Check sheet for the modelled part. Datum: model origin and axes. Units: mm. A direction names the side the tool comes from. Round coordinates to 2 decimals unless told otherwise and drop trailing zeros. Write each loop counter-clockwise with the first axis right and the second up, starting at its lowest first coordinate (ties: lowest second). Pieces come first, ordered by that corner, then holes. Notation, with made-up numbers: (44, 77.5) -> (102, 77.5) arc R17 ccw to (102, 87.5) -> close; hole circle Ø10 at (43, 57.5). An arc over 180 degrees is marked (long way). One line per item, written item: value.
from build123d import *

# Parameters (mm, degrees)
SKETCH1_W                  = 200
SKETCH1_H                  = 54
BOSS_EXTRUDE1_DEPTH        = 75
SHELL1_T                   = 5
BOSS_EXTRUDE2_DEPTH        = 5
BOSS_EXTRUDE3_DEPTH        = 5
SKETCH3_R                  = 1.4
CUT_EXTRUDE1_DEPTH         = 6
BOSS_EXTRUDE4_DEPTH        = 10
SKETCH9_W                  = 45
SKETCH9_H                  = 20
BOSS_EXTRUDE6_DEPTH        = 2
CUT_EXTRUDE2_REACH         = 231.462
SKETCH10_W                 = 12
SKETCH10_H                 = 2
SKETCH11_R                 = 2.3
CUT_EXTRUDE3_DEPTH         = 6
SKETCH13_W                 = 10.5
SKETCH13_H                 = 15
BOSS_EXTRUDE8_DEPTH        = 27
BOSS_EXTRUDE9_DEPTH        = 3.2
CUT_EXTRUDE4_REACH         = 130.496
SKETCH15_R                 = 1.4
CHAMFER8_SIZE              = 0.5
CHAMFER8_OF_MIRROR6_SIZE   = 0.5
CHAMFER3_SIZE              = 40
CHAMFER5_SIZE              = 43
CHAMFER9_SIZE              = 5
CHAMFER10_SIZE             = 2
CHAMFER11_SIZE             = 10
CHAMFER12_SIZE             = 13
CHAMFER13_SIZE             = 4
BOSS_EXTRUDE10_DEPTH       = 3
CHAMFER14_SIZE             = 3
CHAMFER14_OF_MIRROR28_SIZE = 3


# Some blends are built 0.0001 mm under size
with BuildPart() as part:
    # Sketch1 → Boss-Extrude1 (new body)
    with BuildSketch(Plane(origin=(0, 0, 0), x_dir=(1, 0, 0), z_dir=(0, 1, 0))):
        Rectangle(SKETCH1_W, SKETCH1_H)
    extrude(amount=BOSS_EXTRUDE1_DEPTH)

    # Shell1
    shell1_openings = [part.faces().sort_by_distance(p)[0] for p in [
        (0, 75, 0),
    ]]
    offset(amount=SHELL1_T, openings=shell1_openings, kind=Kind.INTERSECTION)

    # Sketch2 → Boss-Extrude2 (add)
    with BuildSketch(Plane(origin=(105, 0, 0), x_dir=(0, 0, -1), z_dir=(1, 0, 0))):
        Polygon((-17, 75), (-6, 86), (6, 86), (17, 75), align=None)
    boss_extrude2 = extrude(amount=-BOSS_EXTRUDE2_DEPTH)

    # Sketch4 → Boss-Extrude3 (add)
    with BuildSketch(Plane(origin=(0, 0, -32), x_dir=(-1, 0, 0), z_dir=(0, 0, -1))):
        Polygon((-80, 75), (-57, 98), (57, 98), (80, 75), align=None)
    boss_extrude3 = extrude(amount=-BOSS_EXTRUDE3_DEPTH)

    # Sketch3 → Cut-Extrude1 (cut)
    with BuildSketch(Plane(origin=(0, 0, -32), x_dir=(-1, 0, 0), z_dir=(0, 0, -1))):
        with Locations((-28, 93)):
            Circle(SKETCH3_R)
        with Locations((-28, 61)):
            Circle(SKETCH3_R)
        with Locations((28, 93)):
            Circle(SKETCH3_R)
        with Locations((28, 61)):
            Circle(SKETCH3_R)
    cut_extrude1 = extrude(amount=-CUT_EXTRUDE1_DEPTH, mode=Mode.SUBTRACT)

    # Mirror4: Boss-Extrude3, Cut-Extrude1 across plane
    add(boss_extrude3.mirror(Plane.XY))
    add(cut_extrude1.mirror(Plane.XY), mode=Mode.SUBTRACT)

    # Mirror5: Boss-Extrude2 across plane
    add(boss_extrude2.mirror(Plane(origin=(0, 0, 0), x_dir=(0, 0, 1), z_dir=(1, 0, 0))))

    # Sketch5 → Boss-Extrude4 (add, symmetric)
    with BuildSketch(Plane.XY):
        Polygon((-100, 75), (-55, 75), (-55, 67), (-100, 22), align=None)
    boss_extrude4 = extrude(amount=BOSS_EXTRUDE4_DEPTH, both=True)

    # Sketch9 → Boss-Extrude6 (add)
    with BuildSketch(Plane(origin=(0, 75, 0), x_dir=(1, 0, 0), z_dir=(0, 1, 0))):
        with Locations((-77.5, 0)):
            Rectangle(SKETCH9_W, SKETCH9_H)
    boss_extrude6 = extrude(amount=BOSS_EXTRUDE6_DEPTH)

    # Sketch10 → Cut-Extrude2 (cut, up to next)
    with BuildSketch(Plane(origin=(-100, 0, 0), x_dir=(0, 0, -1), z_dir=(1, 0, 0)), mode=Mode.PRIVATE) as cut_extrude2_sk1:
        with Locations((0, 76)):
            Rectangle(SKETCH10_W, SKETCH10_H)
    cut_extrude2_tool1 = extrude(cut_extrude2_sk1.sketch, amount=CUT_EXTRUDE2_REACH, mode=Mode.PRIVATE) & part.part
    cut_extrude2 = cut_extrude2_tool1.solids().sort_by_distance((-100, 76, 0))[0]
    add(cut_extrude2, mode=Mode.SUBTRACT)

    # Sketch11 → Cut-Extrude3 (cut)
    with BuildSketch(Plane(origin=(0, 75, 0), x_dir=(1, 0, 0), z_dir=(0, 1, 0))):
        with Locations(Location((-90, 0, 0), (0, 0, 270))):
            Circle(SKETCH11_R)
    cut_extrude3 = extrude(amount=-CUT_EXTRUDE3_DEPTH, mode=Mode.SUBTRACT)

    # Mirror24: Boss-Extrude4, Boss-Extrude6, Cut-Extrude2, Cut-Extrude3 across plane
    add(boss_extrude4.mirror(Plane(origin=(0, 0, 0), x_dir=(0, 0, 1), z_dir=(1, 0, 0))))
    add(boss_extrude6.mirror(Plane(origin=(0, 0, 0), x_dir=(0, 0, 1), z_dir=(1, 0, 0))))
    add(cut_extrude2.mirror(Plane(origin=(0, 0, 0), x_dir=(0, 0, 1), z_dir=(1, 0, 0))), mode=Mode.SUBTRACT)
    add(cut_extrude3.mirror(Plane(origin=(0, 0, 0), x_dir=(0, 0, 1), z_dir=(1, 0, 0))), mode=Mode.SUBTRACT)

    # Sketch13 → Boss-Extrude8 (add, symmetric)
    with BuildSketch(Plane.XY):
        with Locations((35.75, 23.7)):
            Rectangle(SKETCH13_W, SKETCH13_H)
        with Locations((-15.75, 23.7)):
            Rectangle(SKETCH13_W, SKETCH13_H)
    extrude(amount=BOSS_EXTRUDE8_DEPTH, both=True)

    # Sketch14 → Boss-Extrude9 (add)
    with BuildSketch(Plane(origin=(0, 31.2, 0), x_dir=(1, 0, 0), z_dir=(0, 1, 0))):
        with BuildLine():
            Line((-10.5, -27), (-10.5, -9.6))
            Line((-10.5, -9.6), (-15.5, -9.6))
            ThreePointArc((-15.5, -9.6), (-16.914213562, -9.014213562), (-17.5, -7.6))
            Line((-17.5, -7.6), (-17.5, 7.6))
            ThreePointArc((-17.5, 7.6), (-16.914213562, 9.014213562), (-15.5, 9.6))
            Line((-15.5, 9.6), (-10.5, 9.6))
            Line((-10.5, 9.6), (-10.5, 27))
            Line((-10.5, 27), (-21, 27))
            Line((-21, 27), (-21, -27))
            Line((-21, -27), (-10.5, -27))
        make_face()
    boss_extrude9 = extrude(amount=BOSS_EXTRUDE9_DEPTH)

    # Sketch15 → Cut-Extrude4 (cut, up to next)
    with BuildSketch(Plane(origin=(0, 31.2, 0), x_dir=(1, 0, 0), z_dir=(0, 1, 0)), mode=Mode.PRIVATE) as cut_extrude4_sk1:
        with Locations(Location((-14.8, 5, 0), (0, 0, 180))):
            Circle(SKETCH15_R)
    cut_extrude4_tool1 = extrude(cut_extrude4_sk1.sketch, amount=-CUT_EXTRUDE4_REACH, mode=Mode.PRIVATE) & part.part
    # Sketch15 → Cut-Extrude4 (cut, up to next)
    with BuildSketch(Plane(origin=(0, 31.2, 0), x_dir=(1, 0, 0), z_dir=(0, 1, 0)), mode=Mode.PRIVATE) as cut_extrude4_sk2:
        with Locations(Location((-14.8, -5, 0), (0, 0, 180))):
            Circle(SKETCH15_R)
    cut_extrude4_tool2 = extrude(cut_extrude4_sk2.sketch, amount=-CUT_EXTRUDE4_REACH, mode=Mode.PRIVATE) & part.part
    cut_extrude4_1 = cut_extrude4_tool1.solids().sort_by_distance((-14.8, 31.2, -5))[0]
    add(cut_extrude4_1, mode=Mode.SUBTRACT)
    cut_extrude4_2 = cut_extrude4_tool2.solids().sort_by_distance((-14.8, 31.2, 5))[0]
    add(cut_extrude4_2, mode=Mode.SUBTRACT)
    cut_extrude4 = cut_extrude4_1 + cut_extrude4_2  # Cut-Extrude4 as one shape, for the pattern or mirror that repeats it

    # Chamfer8
    chamfer8_edges = [part.edges().sort_by_distance(p)[0] for p in [
        (-13.4, 31.2, -5),
        (-13.4, 31.2, 5),
    ]]
    chamfer(chamfer8_edges, length=CHAMFER8_SIZE)

    # Mirror6: Boss-Extrude9, Cut-Extrude4 across plane
    add(boss_extrude9.mirror(Plane(origin=(10, 0, 0), x_dir=(0, 0, 1), z_dir=(1, 0, 0))))
    add(cut_extrude4.mirror(Plane(origin=(10, 0, 0), x_dir=(0, 0, 1), z_dir=(1, 0, 0))), mode=Mode.SUBTRACT)

    # Chamfer8 of Mirror6
    chamfer8_of_mirror6_edges = [part.edges().sort_by_distance(p)[0] for p in [
        (33.4, 31.2, -5),
        (33.4, 31.2, 5),
    ]]
    chamfer(chamfer8_of_mirror6_edges, length=CHAMFER8_OF_MIRROR6_SIZE)

    # Chamfer3
    # the kernel refuses this chamfer: 40 mm, written as the material it adds along each edge
    with BuildSketch(Plane(origin=(100, 0, 27), x_dir=(0.027495876610586317, 0.9996219169112968, 0), z_dir=(0, 0, -1)), Plane(origin=(-100, 0, -27), x_dir=(-0.027495876610586317, 0.9996219169112968, 0), z_dir=(0, 0, 1))) as chamfer3_piece_1:
        Polygon((CHAMFER3_SIZE * 0.999621916911, -CHAMFER3_SIZE * 0.0274958766106), (-CHAMFER3_SIZE * 0.0274958766106, -CHAMFER3_SIZE * 0.999621916911), (0, 0), align=None)
    extrude(amount=54)

    # Chamfer5
    chamfer5_edges = [part.edges().sort_by_distance(p)[0] for p in [
        (-105, -5, 0),
        (105, -5, 0),
    ]]
    chamfer(chamfer5_edges, length=CHAMFER5_SIZE)

    # Chamfer9
    chamfer9_edges = [part.edges().sort_by_distance(p)[0] for p in [
        (35.75, 16.2, -27),
        (35.75, 16.2, 27),
        (-15.75, 16.2, -27),
        (-15.75, 16.2, 27),
    ]]
    chamfer(chamfer9_edges, length=CHAMFER9_SIZE)

    # Chamfer10
    chamfer10_edges = [part.edges().sort_by_distance(p)[0] for p in [
        (30.5, 22.8, -27),
        (41, 22.8, -27),
        (30.5, 22.8, 27),
        (41, 22.8, 27),
        (-10.5, 22.8, 27),
        (-21, 22.8, 27),
        (-10.5, 22.8, -27),
        (-21, 22.8, -27),
    ]]
    chamfer(chamfer10_edges, length=CHAMFER10_SIZE)

    # Chamfer11
    chamfer11_edges = [part.edges().sort_by_distance(p)[0] for p in [
        (-80, 20, -27),
        (80, 20, -27),
        (-80, 20, 27),
        (80, 20, 27),
    ]]
    chamfer(chamfer11_edges, length=CHAMFER11_SIZE)

    # Chamfer12
    chamfer12_edges = [part.edges().sort_by_distance(p)[0] for p in [
        (-83.5, 16.5, -32),
        (83.5, 16.5, -32),
        (-83.5, 16.5, 32),
        (83.5, 16.5, 32),
    ]]
    chamfer(chamfer12_edges, length=CHAMFER12_SIZE)

    # Chamfer13
    chamfer13_edges = [part.edges().sort_by_distance(p)[0] for p in [
        (-100, 58.5, -10),
        (-100, 58.5, 10),
        (100, 58.5, 10),
        (100, 58.5, -10),
    ]]
    chamfer(chamfer13_edges, length=CHAMFER13_SIZE)

    # Sketch16 → Boss-Extrude10 (add)
    with BuildSketch(Plane(origin=(105, 0, 0), x_dir=(0, 0, -1), z_dir=(1, 0, 0))):
        Polygon((-19, 38), (19, 38), (32, 56.384776311), (32, 75), (17, 75), (6, 86), (-6, 86), (-17, 75), (-32, 75), (-32, 56.384776311), align=None)
    boss_extrude10 = extrude(amount=BOSS_EXTRUDE10_DEPTH)

    # Chamfer14
    chamfer14_edges = [part.edges().sort_by_distance(p)[0] for p in [
        (108, 65.692388155, 32),
        (108, 75, 24.5),
        (108, 80.5, 11.5),
        (108, 86, 0),
        (108, 80.5, -11.5),
        (108, 75, -24.5),
        (108, 65.692388155, -32),
        (108, 47.192388155, -25.5),
        (108, 38, 0),
        (108, 47.192388155, 25.5),
    ]]
    chamfer(chamfer14_edges, length=CHAMFER14_SIZE - 0.0001)  # a hair under: the kernel refuses the full size

    # Mirror28: Boss-Extrude10 across plane
    add(boss_extrude10.mirror(Plane(origin=(0, 0, 0), x_dir=(0, 0, 1), z_dir=(1, 0, 0))))

    # Chamfer14 of Mirror28
    chamfer14_of_mirror28_edges = [part.edges().sort_by_distance(p)[0] for p in [
        (-108, 65.692388155, 32),
        (-108, 75, 24.5),
        (-108, 80.5, 11.5),
        (-108, 86, 0),
        (-108, 80.5, -11.5),
        (-108, 75, -24.5),
        (-108, 65.692388155, -32),
        (-108, 47.192388155, -25.5),
        (-108, 38, 0),
        (-108, 47.192388155, 25.5),
    ]]
    chamfer(chamfer14_of_mirror28_edges, length=CHAMFER14_OF_MIRROR28_SIZE - 0.0001)  # a hair under: the kernel refuses the full size


solid = part.part
Item 1: Tool access check on faces 4 (the flat face through (-1, 0, 0)), 5 (the flat face through (95, 75, 28)), 6 (the flat face through (-98, 57, 12)). Record the directions out of +Z, -Z, +X, -X, +Y, -Y that give a thin tool (end or side, any length) a straight path to the whole face; none if there is none.
Result set:
face 4: none
face 5: +Z, +X, +Y
face 6: +Y
Item 2: Sectioned sample at B-B (x = -32). Enter the section's corners in (y, z).
Result set:
outline: (-5, -32) -> (98, -32) -> (98, -27) -> (0, -27) -> (0, 27) -> (98, 27) -> (98, 32) -> (-5, 32) -> close
Item 3: Sectioned sample at A-A (x = -70). Enter the section's corners in (y, z).
Result set:
outline: (3, -19) -> (21.38, -32) -> (85, -32) -> (85, -27) -> (24.14, -27) -> (10, -17) -> (10, 17) -> (24.14, 27) -> (85, 27) -> (85, 32) -> (21.38, 32) -> (3, 19) -> close; (52, -10) -> (77, -10) -> (77, -6) -> (75, -6) -> (75, 6) -> (77, 6) -> (77, 10) -> (52, 10) -> close
Item 4: Release check for a two-part mould opening along Y. For faces 1 (the flat face through (95, 75, -28)), 2 (the flat face through (-55, 72, 0)), 3 (the flat face through (35.6, 13.7, -24.5)) record: pulls with the +Y half, pulls with the -Y half, needs draft (parallel to the pull), parting line crosses it, or undercut.
Result set:
face 1: pulls with the +Y half
face 2: needs draft
face 3: undercut
Item 5: Depth check by flat-ended pin: pin 1 (16.5 mm diameter, centred on x = -98, z = 26.5, fed in from +Y); pin 2 (3 mm diameter, centred on x = 78.5, z = -5, fed in from -Y); pin 3 (6 mm diameter, centred on x = -90, z = 0, fed in from -Y). Enter the tip coordinate at first touch or a pass-through.
Result set:
pin 1: y = 75
pin 2: y = 10
pin 3: y = 20
Item 6: Material ranges on line 1 along Z through (x, y) = (-71, 76.5); line 2 along X through (y, z) = (72.4, 0); line 3 along Y through (x, z) = (28, 29.65), recorded low to high.
Result set:
line 1: -32 to -27, -10 to -6, 6 to 10, 27 to 32
line 2: -108 to -92.3, -87.7 to -55, 55 to 87.7, 92.3 to 108
line 3: -5 to 59.6, 62.4 to 91.6, 94.4 to 98
Item 7: Sectioned sample at C-C (y = 22.5). State how many separate pieces and enclosed holes the cut face has, then the cut area to 3 significant figures.
Result set:
separate pieces: 1
enclosed holes: 7
area: 3,480 mm^2
